from build123d import *

# Parameters (mm, degrees)
SKETCH1_R           = 1.5
SKETCH1_R_2         = 2.5
SKETCH1_W           = 9
SKETCH1_H           = 4
BOSS_EXTRUDE1_DEPTH = 4


with BuildPart() as part:
    # Sketch1 → Boss-Extrude1 (new body)
    with BuildSketch(Plane.XY):
        with BuildLine():
            Line((55, 39.098584833), (55, 29.098584833))
            ThreePointArc((55, 29.098584833), (54.414213562, 27.684371271), (53, 27.098584833))
            Line((53, 27.098584833), (36.598884751, 27.098584833))
            ThreePointArc((36.598884751, 27.098584833), (32.740210108, 26.722820615), (29.026530651, 25.609647833))
            Line((29.026530651, 25.609647833), (15.772178259, 20.187665872))
            ThreePointArc((15.772178259, 20.187665872), (0.275725932, 27.651148274), (11, 41.098584833))
            Line((11, 41.098584833), (53, 41.098584833))
            ThreePointArc((53, 41.098584833), (54.414213562, 40.512798396), (55, 39.098584833))
        make_face()
        with Locations((38, 36.998584833)):
            Circle(SKETCH1_R, mode=Mode.SUBTRACT)
        with Locations((49.3, 36.998584833)):
            Circle(SKETCH1_R, mode=Mode.SUBTRACT)
        with Locations((11, 30.098584833)):
            Circle(SKETCH1_R_2, mode=Mode.SUBTRACT)
        with Locations((45.5, 32.398584833)):
            Rectangle(SKETCH1_W, SKETCH1_H, mode=Mode.SUBTRACT)
    extrude(amount=BOSS_EXTRUDE1_DEPTH)


solid = part.part
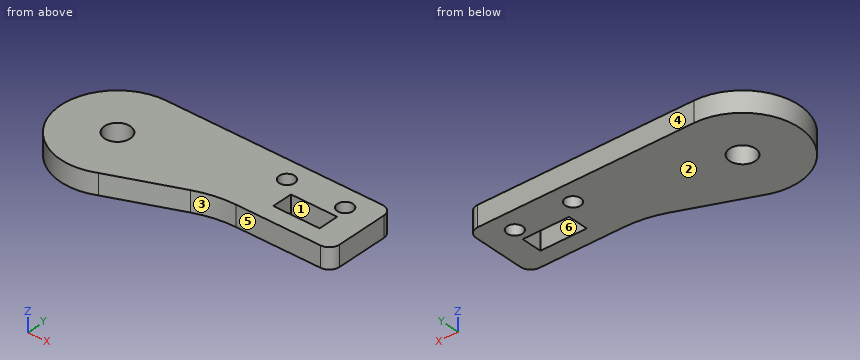
Read the model definition and answer for the solid it produces. Units are mm, in the model's axes. Face numbers are marked on the shaded views. A direction names the side the tool comes from. Give positions to 0.01 mm unless a question says otherwise; leave off trailing zeros. Write each loop counter-clockwise with the first axis right and the second up, starting at its lowest first coordinate (ties: lowest second). Pieces come first, ordered by that corner, then holes. Notation, with made-up numbers: (18.25, 4) - (67.25, 4) arc R8 cw to (67.25, 9) - close; hole circle Ø3 at (6, 61). An arc over 180 degrees is marked (long way). Return JSON: item names as keys, results as strings.
Q1. A cutting plane is placed at B-B, the plane x = 49.3. Determine the outline of the cut face in (y, z), and give its area (3 significant figures).
Reply:
{"outline": "(27.1, 0) - (30.4, 0) - (30.4, 4) - (27.1, 4) - close; (34.4, 0) - (35.5, 0) - (35.5, 4) - (34.4, 4) - close; (38.5, 0) - (41.1, 0) - (41.1, 4) - (38.5, 4) - close", "area": "28.0 mm²"}
Q2. A cutting plane is placed at C-C, the plane y = 36.5. Determine the outline of the cut face in (x, z), and give its area (3 significant figures).
Reply:
{"outline": "(2.05, 0) - (36.59, 0) - (36.59, 4) - (2.05, 4) - close; (39.41, 0) - (47.89, 0) - (47.89, 4) - (39.41, 4) - close; (50.71, 0) - (55, 0) - (55, 4) - (50.71, 4) - close", "area": "189 mm²"}
Q3. For the marked faces 4, 5 and 6, determine the directions among +Z, -Z, +X, -X, +Y, -Y from which every point of the face is accessible in a straight line to the end or side of a thin tool.
Reply:
{"face 4": "+Z, -Z, +X, -X, +Y", "face 5": "+Z, -Z, +X, -Y", "face 6": "+Z, -Z"}
Q4. Given P1, Ø2, axis at x = 46.5, z = 2.5, coming from the -Y side; P2, Ø1, axis at x = 17, z = 3, coming from the -Y side; P3, Ø1.2, axis at y = 31.5, z = 2.5, coming from the -X side; P4, Ø2.5, axis at x = 38, y = 37, coming from the +Z side, each flat-ended and moving along its own axis, determine where each tip first touches the part or whether it passes through.
Reply:
{"P1": "y = 27.1", "P2": "y = 20.49", "P3": "x = 0.03", "P4": "through"}
Q5. For a pull along X with two mould halves and no side action, classify the marked faces 1, 2 and 3 as released by +X, released by -X, zero draft, split by the parting line, or undercut.
Reply:
{"face 1": "undercut", "face 2": "zero draft", "face 3": "released by +X"}
Q6. A cutting plane is placed at A-A, the plane x = 38. Determine the outline of the cut face in (y, z).
Reply:
{"outline": "(27.1, 0) - (35.5, 0) - (35.5, 4) - (27.1, 4) - close; (38.5, 0) - (41.1, 0) - (41.1, 4) - (38.5, 4) - close"}
Q7. A cutting plane is placed at D-D, the plane z = 1.7. Determine the outline of the cut face in (x, y).
Reply:
{"outline": "(11, 41.1) arc R11 ccw (long way) to (15.77, 20.19) - (29.03, 25.61) arc R20 cw to (36.6, 27.1) - (53, 27.1) arc R2 ccw to (55, 29.1) - (55, 39.1) arc R2 ccw to (53, 41.1) - close; hole circle Ø5 at (11, 30.1); hole circle Ø3 at (38, 37); hole (41, 30.4) - (50, 30.4) - (50, 34.4) - (41, 34.4) - close; hole circle Ø3 at (49.3, 37)"}
Q8. Consider line 1 along Y through (x, z) = (49.3, 2.65); line 2 along X through (y, z) = (36, 3.7); line 3 along X through (y, z) = (36.5, 0.6). Determine where each line is inside the solid, lowest interval first. Write a range as [from, to].
Reply:
{"line 1": "[27.1, 30.4], [34.4, 35.5], [38.5, 41.1]", "line 2": "[1.72, 36.88], [39.12, 48.18], [50.42, 55]", "line 3": "[2.05, 36.59], [39.41, 47.89], [50.71, 55]"}
